The drawing under review shows one solid part. Ordinate dimensions are in mm from its lowest x, y, z. A direction names the side the tool comes from. Coordinates: 2 decimals unless noted, no trailing zeros. Order: outer loops, then holes, each group sorted by start corner. A loop starts at its lowest first (then second) coordinate and runs counter-clockwise, first axis right, second up.
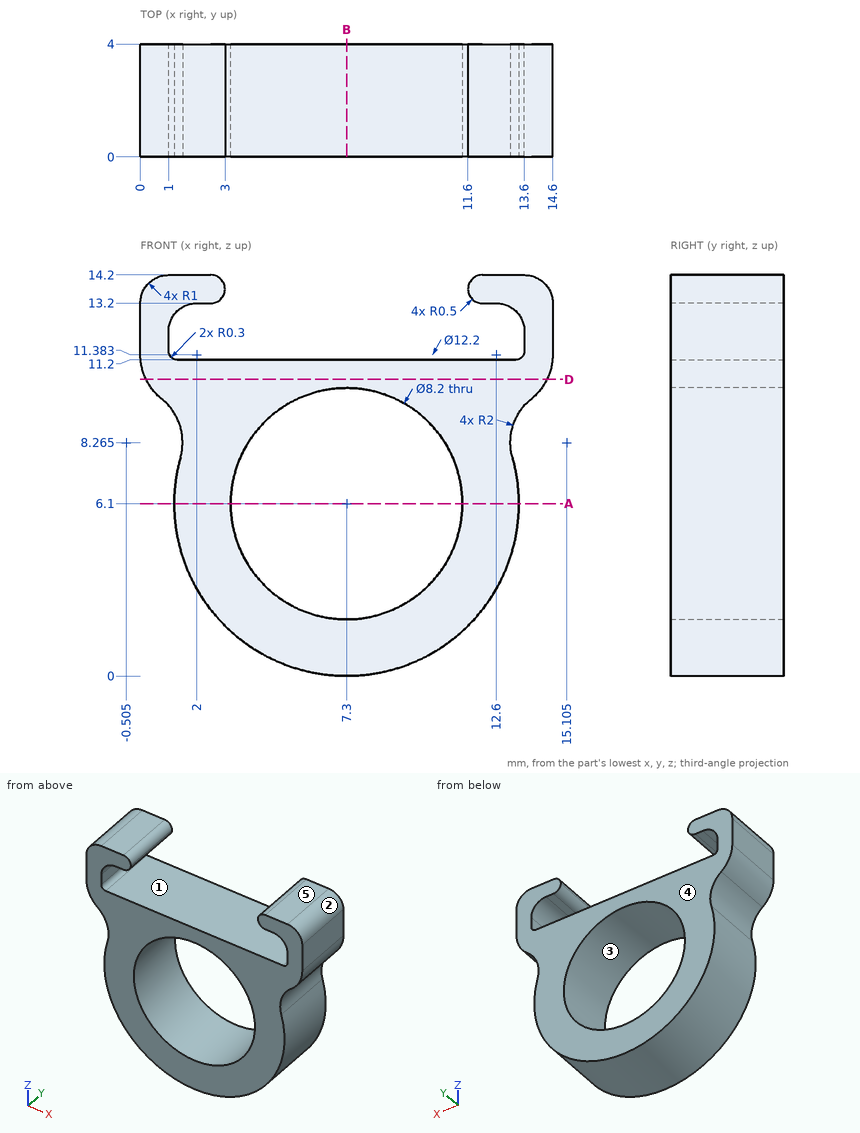
(1) We need section D-D, the plane z = 10.5. Write out the cut boundary in (x, y) (1 decimal).
A:
outline: (0.2, 0) - (14.4, 0) - (14.4, 4) - (0.2, 4) - close
(2) We need section B-B, the plane x = 7.3. Write out the cut boundary in (y, z).
A:
outline: (0, 0) - (4, 0) - (4, 2) - (0, 2) - close; (0, 10.2) - (4, 10.2) - (4, 11.2) - (0, 11.2) - close
(3) Wall thickness on probe 1 along Z at (x, y) = (7.3, 2.2); probe 2 along X at (y, z) = (2.95, 12); probe 3 along X at (y, z) = (3.1, 6.1): over which ranges is each line inside the solid? List them lowest first.
A:
probe 1: z = 0 to 2, 10.2 to 11.2
probe 2: x = 0 to 1, 13.6 to 14.6
probe 3: x = 1.2 to 3.2, 11.4 to 13.4
(4) We need section A-A, the plane z = 6.1. Write out the cut boundary in (x, y).
A:
outline: (1.2, 0) - (3.2, 0) - (3.2, 4) - (1.2, 4) - close; (11.4, 0) - (13.4, 0) - (13.4, 4) - (11.4, 4) - close
(5) For pin 1 Ø1.5 at (y, z) = (0.5, 2) entering from +X; pin 2 Ø2 at (x, y) = (8.5, 2.5) entering from +Z; pin 3 Ø0.6 at (x, y) = (2.5, 3) entering from -Z, all flat-tipped, find the tip position at first contact; note any pin that passes through.
A:
pin 1: stops at x = 12.4
pin 2: stops at z = 11.2
pin 3: stops at z = 1.98
(6) Machinability: for the marked faces 1 and 2, which of the approach directions +Z, -Z, +X, -X, +Y, -Y give a long, thin tool a straight path to every point of the face, cutting with its end or side? Answer none if there is none.
A:
face 1: +Y, -Y
face 2: +Z, +X, +Y, -Y
(7) Draft analysis for pull direction Z (two halves, no side actions). For the marked faces 3, 4 and 5, state which applies: released by +Z, released by -Z, zero draft, split by the parting line, or undercut.
A:
face 3: undercut
face 4: zero draft
face 5: released by +Z
